from build123d import *

# Parameters (mm, degrees)
BOSS_EXTRUDE2_DEPTH = 5
FILLET1_R           = 0.5


with BuildPart() as part:
    # Sketch1 → Boss-Extrude2 (new body)
    with BuildSketch(Plane(origin=(0, 0, 0), x_dir=(1, 0, 0), z_dir=(0, 1, 0))):
        Polygon((46.062322946, -39.44276686), (15.062322946, -39.44276686), (15.062322946, -49.44276686), (17.062322946, -49.44276686), (17.062322946, -41.44276686), (37.062322946, -41.44276686), (37.062322946, -66.44276686), (17.062322946, -66.44276686), (17.062322946, -58.44276686), (15.062322946, -58.44276686), (15.062322946, -68.44276686), (46.062322946, -68.44276686), align=None)
        Polygon((44.062322946, -56.44276686), (39.062322946, -56.44276686), (39.062322946, -51.44276686), (44.062322946, -51.44276686), (44.062322946, -52.94276686), (42.062322946, -52.94276686), (42.062322946, -54.94276686), (44.062322946, -54.94276686), align=None, mode=Mode.SUBTRACT)
    extrude(amount=BOSS_EXTRUDE2_DEPTH)

    # Fillet1
    fillet1_edges = [part.edges().sort_by_distance(p)[0] for p in [
        (41.562322946, 5, 51.44276686),
        (44.062322946, 5, 52.19276686),
        (16.062322946, 0, 49.44276686),
        (43.062322946, 5, 52.94276686),
        (46.062322946, 0, 53.94276686),
        (30.562322946, 0, 68.44276686),
        (17.062322946, 0, 62.44276686),
        (27.062322946, 0, 66.44276686),
        (37.062322946, 0, 53.94276686),
        (42.062322946, 5, 53.94276686),
        (27.062322946, 0, 41.44276686),
        (17.062322946, 0, 45.44276686),
        (44.062322946, 0, 52.19276686),
        (41.562322946, 0, 51.44276686),
        (39.062322946, 0, 53.94276686),
        (41.562322946, 0, 56.44276686),
        (17.062322946, 2.5, 49.44276686),
        (15.062322946, 2.5, 49.44276686),
        (46.062322946, 2.5, 39.44276686),
        (46.062322946, 2.5, 68.44276686),
        (15.062322946, 2.5, 68.44276686),
        (17.062322946, 2.5, 58.44276686),
        (17.062322946, 2.5, 66.44276686),
        (37.062322946, 2.5, 41.44276686),
        (17.062322946, 5, 45.44276686),
        (17.062322946, 2.5, 41.44276686),
        (44.062322946, 2.5, 51.44276686),
        (39.062322946, 2.5, 51.44276686),
        (39.062322946, 2.5, 56.44276686),
        (27.062322946, 5, 41.44276686),
        (37.062322946, 5, 53.94276686),
        (41.562322946, 5, 56.44276686),
        (27.062322946, 5, 66.44276686),
        (44.062322946, 0, 55.69276686),
        (44.062322946, 5, 55.69276686),
        (17.062322946, 5, 62.44276686),
        (44.062322946, 2.5, 54.94276686),
        (16.062322946, 5, 58.44276686),
        (15.062322946, 5, 63.44276686),
        (42.062322946, 2.5, 54.94276686),
        (43.062322946, 5, 54.94276686),
        (43.062322946, 0, 54.94276686),
        (30.562322946, 5, 68.44276686),
        (46.062322946, 5, 53.94276686),
        (30.562322946, 5, 39.44276686),
        (39.062322946, 5, 53.94276686),
        (15.062322946, 5, 44.44276686),
        (16.062322946, 5, 49.44276686),
    ]]
    fillet(fillet1_edges, radius=FILLET1_R)


solid = part.part
Geometry: final body of the model. Coordinates: model frame, mm. A direction names the side the tool comes from. Coordinates: 2 decimals unless noted, no trailing zeros. Loops run counter-clockwise (first coordinate to the right, second up) from the corner with the lowest first, then second, coordinate; pieces in that order, holes last. Notation, with made-up numbers: (65.25, -32.75) - (70.25, -32.75) arc R17 cw to (70.25, -5.75) - close; hole circle Ø11 at (31.25, 4). An arc over 180 degrees is marked (long way). Put each result on its own line as item: value. Start each with the question number.
Q1. Line query: line 1 (X direction, y = 4.5, z = 56); line 2 (Z direction, x = 19, y = 3.25); line 3 (Z direction, x = 42.5, y = 1.7). Output: solid intervals per line, ascending.
Q2. Pull-direction query (Z, two-part tool) for faces 1 (the flat face through (43, 2, 54.943)), 2 (the flat face through (15.062, 2, 63)), 3 (the flat face through (30, 2, 68.443)); classes: released by +Z, released by -Z, zero draft, split by the parting line, or undercut.
Q3. Pin query (flat end, axial travel): pin 1 Ø10 at (x, z) = (41, 55.5) entering from +Y; pin 2 Ø0.5 at (y, z) = (3.5, 52.5) entering from -X; pin 3 Ø2 at (x, z) = (34.5, 47) entering from +Y. Return the tip coordinate at first contact, or that it passes through.
Q4. Set-up query: faces 4 (the flat face through (16, 2, 49.443)), 5 (the flat face through (38, 5, 54)), 6 (the flat face through (37.062, 2, 54)). Return all of +Z, -Z, +X, -X, +Y, -Y with unobstructed straight access to the full face (end or side cutting, diameter ignored); none if empty.
Q5. Cut plane A-A, the plane z = 60. Return loops of the section in (x, y), and give its area (3 significant figures).
Q6. Cut plane B-B, the plane x = 28. Return loops of the section in (y, z).
Filled sheet:
1. line 1: 37.06 to 39.07, 44.06 to 46.06
1. line 2: 39.44 to 41.44, 66.44 to 68.44
1. line 3: 39.44 to 51.44, 52.94 to 54.94, 56.44 to 68.44
2. face 1: undercut
2. face 2: zero draft
2. face 3: released by +Z
3. pin 1: y = 5
3. pin 2: x = 37.06
3. pin 3: through
4. face 4: -X, +Y, -Y
4. face 5: +Z, -Z, +X, -X, +Y
4. face 6: +Y, -Y
5. outline: (15.06, 0) - (16.56, 0) arc R0.5 ccw to (17.06, 0.5) - (17.06, 4.5) arc R0.5 ccw to (16.56, 5) - (15.56, 5) arc R0.5 ccw to (15.06, 4.5) - close; (37.06, 0.5) arc R0.5 ccw to (37.56, 0) - (45.56, 0) arc R0.5 ccw to (46.06, 0.5) - (46.06, 4.5) arc R0.5 ccw to (45.56, 5) - (37.56, 5) arc R0.5 ccw to (37.06, 4.5) - close
5. area: 54.6 mm²
6. outline: (0, 39.44) - (4.5, 39.44) arc R0.5 ccw to (5, 39.94) - (5, 40.94) arc R0.5 ccw to (4.5, 41.44) - (0.5, 41.44) arc R0.5 ccw to (0, 40.94) - close; (0, 66.94) arc R0.5 ccw to (0.5, 66.44) - (4.5, 66.44) arc R0.5 ccw to (5, 66.94) - (5, 67.94) arc R0.5 ccw to (4.5, 68.44) - (0.5, 68.44) arc R0.5 ccw to (0, 67.94) - close
